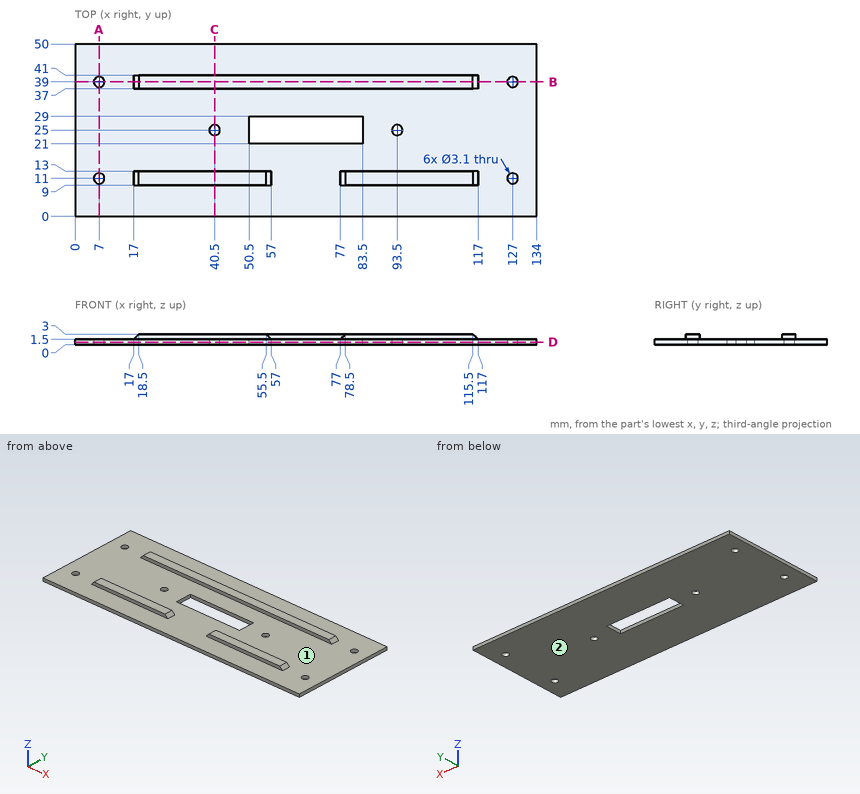
The figure shows three views and two pictorial views of one solid part (mm, origin at its lowest corner). Answer the questions. Round coordinates to 2 decimals unless told otherwise and drop trailing zeros. Order: outer loops, then holes, each group sorted by start corner. A loop starts at its lowest first (then second) coordinate and runs counter-clockwise, first axis right, second up.
Q1. A cutting plane is placed at A-A, the plane x = 7. Determine the outline of the cut face in (y, z).
Solution:
outline: (0, 0) - (9.45, 0) - (9.45, 1.5) - (0, 1.5) - close; (12.55, 0) - (37.45, 0) - (37.45, 1.5) - (12.55, 1.5) - close; (40.55, 0) - (50, 0) - (50, 1.5) - (40.55, 1.5) - close
Q2. A cutting plane is placed at B-B, the plane y = 39. Count the separate pieces of the cut face and the enclosed holes in it.
Solution:
separate pieces: 3
enclosed holes: 0
Q3. Find the intervals of material crossed by line 1 along Y through (x, z) = (127, 0.3); line 2 along X through (y, z) = (27, 0.5); line 3 along Y through (x, z) = (104, 2.6), in increasing order.
Solution:
line 1: y = 0 to 9.45, 12.55 to 37.45, 40.55 to 50
line 2: x = 0 to 50.5, 83.5 to 134
line 3: y = 9 to 13, 37 to 41
Q4. A cutting plane is placed at C-C, the plane x = 40.5. Determine the outline of the cut face in (y, z).
Solution:
outline: (0, 0) - (23.45, 0) - (23.45, 1.5) - (13, 1.5) - (13, 3) - (9, 3) - (9, 1.5) - (0, 1.5) - close; (26.55, 0) - (50, 0) - (50, 1.5) - (41, 1.5) - (41, 3) - (37, 3) - (37, 1.5) - (26.55, 1.5) - close
Q5. A cutting plane is placed at D-D, the plane z = 0.75. Determine the outline of the cut face in (x, y), then the cut area to 3 significant figures.
Solution:
outline: (0, 0) - (134, 0) - (134, 50) - (0, 50) - close; hole circle Ø3.1 at (7, 11); hole circle Ø3.1 at (7, 39); hole circle Ø3.1 at (40.5, 25); hole (50.5, 21) - (83.5, 21) - (83.5, 29) - (50.5, 29) - close; hole circle Ø3.1 at (93.5, 25); hole circle Ø3.1 at (127, 11); hole circle Ø3.1 at (127, 39)
area: 6,390 mm2
Q6. Given pin 1 Ø1.9 at (x, y) = (40.5, 25) entering from -Z; pin 2 Ø4 at (x, y) = (57.5, 29) entering from +Z; pin 3 Ø0.5 at (x, z) = (32.5, 2.5) entering from +Y, each flat-ended and moving along its own axis, determine where each tip first touches the part or whether it passes through.
Solution:
pin 1: passes through
pin 2: stops at z = 1.5
pin 3: stops at y = 41
Q7. The mould has two halves that part along Y. Classify the marked faces 1 and 2: pulls with the +Y half, pulls with the -Y half, needs draft (parallel to the pull), parting line crosses it, or undercut.
Solution:
face 1: undercut
face 2: needs draft
